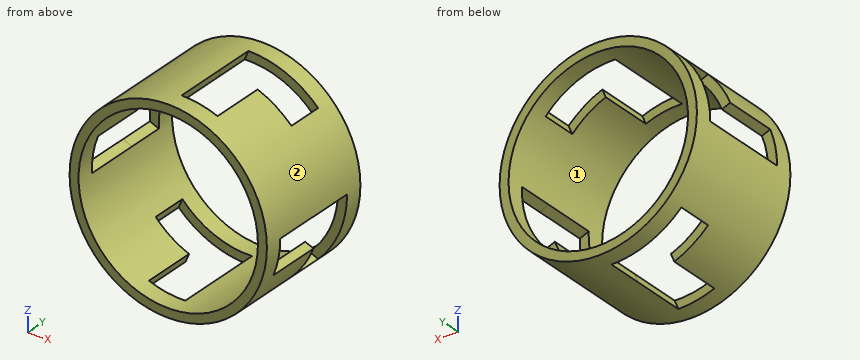
from build123d import *

# Parameters (mm, degrees)
F0_R     = 34.925
F0_R_2   = 31.75
F1_DEPTH = 44.45
F5_DEPTH = 12.7
F8_DEPTH = 19.05


with BuildPart() as f1:
    # F0 (on Front) → F1 (new body)
    with BuildSketch(Plane.XZ):
        Circle(F0_R)
        Circle(F0_R_2, mode=Mode.SUBTRACT)
    extrude(amount=F1_DEPTH)

    # F4 (on offset) → F5 (cut)
    with BuildSketch(Plane.XZ.offset(6.35)):
        Polygon((-29.058365, -2.43004), (-18.829069, 22.265665), (-27.629022, 25.910724), (-37.858318, 1.21502), align=None)
        Polygon((25.910724, 27.629022), (1.21502, 37.858318), (-2.43004, 29.058365), (22.265665, 18.829069), align=None)
        Polygon((29.058365, 2.43004), (18.829069, -22.265665), (27.629022, -25.910724), (37.858318, -1.21502), align=None)
        Polygon((2.43004, -29.058365), (-22.265665, -18.829069), (-25.910724, -27.629022), (-1.21502, -37.858318), align=None)
    extrude(amount=F5_DEPTH, mode=Mode.SUBTRACT)

    # F7 (on offset) → F8 (cut)
    with BuildSketch(Plane.XZ.offset(19.05)):
        Polygon((0, 34.925), (-2.430039, 29.058366), (9.303231, 24.198287), (12.94829, 32.998238), (1.21502, 37.858318), align=None)
        Polygon((-34.925, 0), (-29.058366, -2.430039), (-24.198287, 9.303231), (-32.998238, 12.94829), (-37.858318, 1.21502), align=None)
        Polygon((0, -34.925), (2.430039, -29.058366), (-9.303231, -24.198287), (-12.94829, -32.998238), (-1.21502, -37.858318), align=None)
        Polygon((34.925, 0), (29.058366, 2.430039), (24.198287, -9.303231), (32.998238, -12.94829), (37.858318, -1.21502), align=None)
    extrude(amount=F8_DEPTH, mode=Mode.SUBTRACT)


solid = f1.part
The model under review builds one solid part; all positions refer to its coordinate system, in mm. Face numbers are marked on the shaded views. Give positions to 0.01 mm unless a question says otherwise; leave off trailing zeros. Order: outer loops, then holes, each group sorted by start corner. A loop starts at its lowest first (then second) coordinate and runs counter-clockwise, first axis right, second up. Notation, with made-up numbers: M -31.5,-9.75 L -0.5,-9.75 A24 cw -0.5,19.25 Z; hole C 79,-11 d10. An arc over 180 degrees is marked long. One line per question, with ' | ' between items. Start each with the question number.
1) Consider section B-B, the plane x = -3.5. Give the boundary of the cut face in (y, z).
2) Consider section D-D, the plane y = -31. Give the boundary of the cut face in (x, z) (3 decimals).
3) Consider section C-C, the plane z = -9. Give the boundary of the cut face in (x, y).
4) Clearance check with flat-ended pins moving along their axes: P1, Ø1.5, axis at y = -25.5, z = -19, coming from the -X side; P2, Ø8, axis at y = -9.5, z = -4.5, coming from the +X side; P3, Ø5, axis at y = -34.5, z = 23.5, coming from the +X side. State where each tip first meets the part, or that it passes through.
5) Consider section A-A, the plane y = -13. Give the boundary of the cut face in (x, z) (3 decimals).
6) Wall thickness on L1, parallel to X at y = -34, z = -17.5; L2, parallel to X at y = -23.5, z = 28.5; L3, parallel to Z at x = -8.5, y = -2: over which ranges is each line inside the solid? List them lowest first. Write a range as from..to.
7) Mouldability with a two-part tool opening along X and no side actions: class the marked faces 1 and 2 as pulls with the +X half, pulls with the -X half, needs draft (parallel to the pull), parting line crosses it, or undercut.
Found:
1) outline: M -44.45,-34.75 L -38.1,-34.75 L -38.1,-31.56 L -44.45,-31.56 Z; M -44.45,31.56 L 0,31.56 L 0,34.75 L -44.45,34.75 Z; M -6.35,-34.75 L 0,-34.75 L 0,-31.56 L -6.35,-31.56 Z
2) outline: M -34.925,0 A34.925 ccw -12.748,-32.515 L -11.533,-29.581 A31.75 cw -31.722,-1.327 Z; M -32.515,12.748 L -29.581,11.533 A31.75 cw -1.327,31.722 L 0,34.925 A34.925 ccw Z; M 0,-34.925 A34.925 ccw 32.515,-12.748 L 29.581,-11.533 A31.75 cw 1.327,-31.722 Z; M 11.533,29.581 A31.75 cw 31.722,1.327 L 34.925,0 A34.925 ccw 12.748,32.515 Z
3) outline: M -33.75,-44.45 L -30.45,-44.45 L -30.45,0 L -33.75,0 Z; M 30.45,-44.45 L 33.75,-44.45 L 33.75,-38.1 L 30.45,-38.1 Z; M 30.45,-6.35 L 33.75,-6.35 L 33.75,0 L 30.45,0 Z
4) P1: stops at x = -29.78 | P2: stops at x = 34.87 | P3: stops at x = 27.91
5) outline: M -34.925,0 A34.925 ccw -24.696,-24.696 L -23.369,-21.493 A31.75 cw -31.722,-1.327 Z; M -24.696,24.696 L -21.493,23.369 A31.75 cw -1.327,31.722 L 0,34.925 A34.925 ccw Z; M 0,-34.925 A34.925 ccw 24.696,-24.696 L 21.493,-23.369 A31.75 cw 1.327,-31.722 Z; M 23.369,21.493 A31.75 cw 31.722,1.327 L 34.925,0 A34.925 ccw 24.696,24.696 Z
6) L1: x = -30.22..-26.49, 26.49..30.22 | L2: x = -20.19..-13.99, 13.99..20.19 | L3: z = -33.87..-30.59, 30.59..33.87
7) face 1: undercut | face 2: parting line crosses it
